The listing builds one solid part. Answer for the finished solid, in the listing's coordinates (mm). Round coordinates to 2 decimals unless told otherwise and drop trailing zeros. Write each loop counter-clockwise with the first axis right and the second up, starting at its lowest first coordinate (ties: lowest second). Pieces come first, ordered by that corner, then holes. Notation, with made-up numbers: (-24, 62.5) - (19, 62.5) arc R8 cw to (19, 68.5) - close; hole circle Ø3 at (-33, 6.25). An arc over 180 degrees is marked (long way). Return JSON: item names as keys, results as strings. Group by question number.
(1) Section D-D, the plane y = 75 is taken. Write down the section's boundary in (x, z).
(2) Section A-A, the plane x = 0 is taken. Write down the section's boundary in (y, z).
(3) Find the intervals of material crossed by line 1 along X through (y, z) = (9.05, -0.25); line 2 along X through (y, z) = (1.75, 0); line 3 along Y through (x, z) = (-1.5, -3.25), in increasing order. Write a range as [from, to].
(4) Section B-B, the plane z = 0 is taken. Write down the section's boundary in (x, y).
(5) Section C-C, the plane y = 9.05 is taken. Write down the section's boundary in (x, z), then the cut area to 3 significant figures.
(6) Each of these flat-tipped pins is pushed along its axis until it touches: pin 1 (3 mm diameter, centred on x = 0, z = 0, fed in from -Y); pin 2 (1.5 mm diameter, centred on y = 87, z = -5.5, fed in from +X); pin 3 (3 mm diameter, centred on y = 43.5, z = -7.5, fed in from -X). Where does it stop, or does it pass through?
```python
from build123d import *

# Parameters (mm, degrees)
SKETCH1_R           = 10
BOSS_EXTRUDE1_DEPTH = 178.8
CHAMFER1_SIZE       = 1
SKETCH2_R           = 3.1
CUT_EXTRUDE1_DEPTH  = 155
SKETCH_1_R          = 2.5
CUT_EXTRUDE_1_DEPTH = 10


with BuildPart() as part:
    # Sketch1 → Boss-Extrude1 (new body)
    with BuildSketch(Plane(origin=(0, 0, 0), x_dir=(1, 0, 0), z_dir=(0, 1, 0))):
        with Locations(Location((0, 0, 0), (0, 0, 90))):
            Circle(SKETCH1_R)
    extrude(amount=BOSS_EXTRUDE1_DEPTH)

    # Chamfer1
    chamfer1_edges = [part.edges().sort_by_distance(p)[0] for p in [
        (0, 0, 10),
    ]]
    chamfer(chamfer1_edges, length=CHAMFER1_SIZE)

    # Sketch2 → Cut-Extrude1 (cut)
    with BuildSketch(Plane(origin=(0, 0, -10), x_dir=(-1, 0, 0), z_dir=(0, 0, -1))):
        with Locations((0, 9.05)):
            Circle(SKETCH2_R)
    extrude(amount=-CUT_EXTRUDE1_DEPTH, mode=Mode.SUBTRACT)

    # 草图1 → 切除-拉伸1 (cut)
    with BuildSketch(Plane.XZ):
        with Locations(Location((0, 0, 0), (0, 0, 270))):
            Circle(SKETCH_1_R)
    extrude(amount=-CUT_EXTRUDE_1_DEPTH, mode=Mode.SUBTRACT)


solid = part.part
```
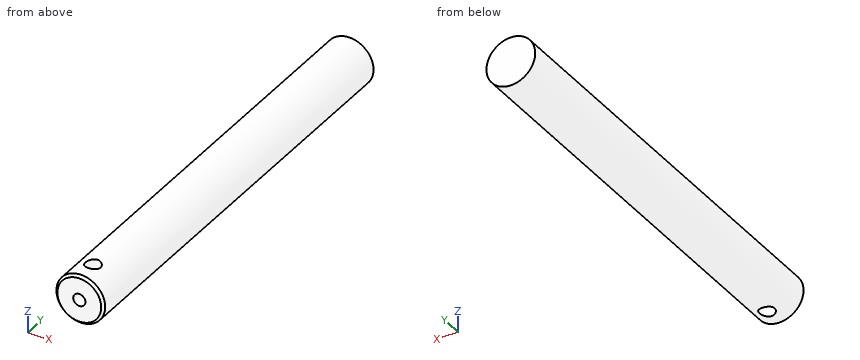
Working result:
{
 "1": {"outline": "circle Ø20 at (0, 0)"},
 "2": {"outline": "(0, -9) - (1, -10) - (5.95, -10) - (5.95, -2.5) - (0, -2.5) - close; (0, 2.5) - (5.95, 2.5) - (5.95, 10) - (1, 10) - (0, 9) - close; (12.15, -10) - (178.8, -10) - (178.8, 10) - (12.15, 10) - close"},
 "3": {"line 1": "x = [-10, -3.1], [3.1, 10]", "line 2": "x = [-10, -2.5], [2.5, 10]", "line 3": "y = [0, 6.34], [11.76, 178.8]"},
 "4": {"outline": "(-10, 1) - (-9, 0) - (-2.5, 0) - (-2.5, 7.22) arc R3.1 cw (long way) to (2.5, 7.22) - (2.5, 0) - (9, 0) - (10, 1) - (10, 178.8) - (-10, 178.8) - close"},
 "5": {"outline": "(-3.1, -9.51) - (-3.1, 9.51) arc R10 ccw to start; (3.1, -9.51) arc R10 ccw to (3.1, 9.51) - close", "area": "192 mm^2"},
 "6": {"pin 1": "stops at y = 11.76", "pin 2": "stops at x = 8.8", "pin 3": "stops at x = -8"}
}
